from build123d import *

# Parameters (mm, degrees)
CHAMFER_1_SIZE         = 0.5
EXTRUDE_1649_DEPTH     = 5.5
SKETCH_6_R             = 8
CUT_EXTRUDE_1797_DEPTH = 0.5
SKETCH_9_R             = 2.5
EXTRUDE_1978_DEPTH     = 3
HOLE_WIZARD_M2_5_D     = 2.5


with BuildPart() as part:
    # Эскиз2 → Revolve 1260 (revolve)
    with BuildSketch(Plane.XY):
        Polygon((0, 4.5), (-9.5, 4.5), (-9.5, -1.5), (-6, -1.5), (-6, 0), (0, 0), align=None)
    revolve(axis=Axis((0, 4.5, 0), (0, -1, 0)))

    # Фаска1
    chamfer_1_edges = [part.edges().sort_by_distance(p)[0] for p in [
        (9.5, 4.5, 0),
    ]]
    chamfer(chamfer_1_edges, length=CHAMFER_1_SIZE)

    # Эскиз8 → Extrude 1649 (add)
    with BuildSketch(Plane.XZ):
        with BuildLine():
            Line((-1.175, 3.175), (1.175, 3.175))
            ThreePointArc((1.175, 3.175), (2.589213562, 2.589213562), (3.175, 1.175))
            Line((3.175, 1.175), (3.175, -1.175))
            ThreePointArc((3.175, -1.175), (2.589213562, -2.589213562), (1.175, -3.175))
            Line((1.175, -3.175), (-1.175, -3.175))
            ThreePointArc((-1.175, -3.175), (-2.589213562, -2.589213562), (-3.175, -1.175))
            Line((-3.175, -1.175), (-3.175, 1.175))
            ThreePointArc((-3.175, 1.175), (-2.589213562, 2.589213562), (-1.175, 3.175))
        make_face()
    extrude(amount=EXTRUDE_1649_DEPTH)

    # Эскиз6 → Cut-Extrude 1797 (cut)
    with BuildSketch(Plane(origin=(0, 4.5, 0), x_dir=(1, 0, 0), z_dir=(0, 1, 0))):
        with Locations(Location((0, 0, 0), (0, 0, 180))):
            Circle(SKETCH_6_R)
    extrude(amount=-CUT_EXTRUDE_1797_DEPTH, mode=Mode.SUBTRACT)

    # Эскиз9 → Extrude 1978 (add)
    with BuildSketch(Plane.XZ.offset(5.5)):
        Circle(SKETCH_9_R)
    extrude(amount=EXTRUDE_1978_DEPTH)

    # Отверстие M2,5 (through all)
    with Locations(Plane(origin=(0, -8.5, 0), x_dir=(-1, 0, 0), z_dir=(0, -1, 0))):
        with Locations((0, 0)):
            Hole(HOLE_WIZARD_M2_5_D / 2)


solid = part.part
The listing builds one solid part. Answer for the finished solid, in the listing's coordinates (mm). A direction names the side the tool comes from. Round coordinates to 2 decimals unless told otherwise and drop trailing zeros. Order: outer loops, then holes, each group sorted by start corner. A loop starts at its lowest first (then second) coordinate and runs counter-clockwise, first axis right, second up. Notation, with made-up numbers: (37, -9.75) -> (88, -9.75) arc R36 cw to (88, 28.25) -> close; hole circle Ø8 at (-16, 57). An arc over 180 degrees is marked (long way). Write each question's results on one line, items separated by ' | '. Start each with the question number.
Q1. Find section D-D (y = -3.5). Determine the outline of the cut face in (x, z) (3 decimals), then the cut area to 3 significant figures.
Q2. Find section B-B (x = 0). Determine the outline of the cut face in (y, z) (3 decimals).
Q3. Straight lines are drawn through the part: probe 1 along Z at (x, y) = (0, -0.75) (3 decimals); probe 2 along Z at (x, y) = (0, -2.25) (3 decimals); probe 3 along Y at (x, z) = (-6.25, -1). For each, find the intervals that lie inside material, in ascending order. Write a range as from..to.
Q4. Find section C-C (z = 0). Determine the outline of the cut face in (x, y) (3 decimals).
Q5. Find section A-A (y = -1). Determine the outline of the cut face in (x, z) (3 decimals), then the cut area to 3 significant figures.
Q6. The mould has two halves that part along X. Classify faces 4 (the cylindrical face through (2.605, -2.712, -2.574)), 5 (the flat face through (0, -3, 3.175)), 6 (the flat face through (-1, -8.5, -1)), 7 (the cylindrical face through (-4.38, 1.21, 8.43)): pulls with the +X half, pulls with the -X half, needs draft (parallel to the pull), parting line crosses it, or undercut.
Q7. Which of the six approach directions +Z, -Z, +X, -X, +Y, -Y give full straight-line access (tool end or side, diameter ignored) to faces 1 (the cylindrical face through (-0.27, -2.16, 1.22)), 2 (the flat face through (0.1, -1.5, 6.2)), 3 (the flat face through (-2, 4, 0))?
Q8. Each of these flat-tipped pins is pushed along its axis until it touches: pin 1 (1 mm diameter, centred on x = 4.5, y = -6.5, fed in from -Z); pin 2 (5 mm diameter, centred on x = 1.5, z = 3.5, fed in from +Y); pin 3 (10 mm diameter, centred on x = -7, z = 3, fed in from -Y). Where does it stop, or does it pass through?
Worked answers:
1) outline: (-3.175, -1.175) arc R2 ccw to (-1.175, -3.175) -> (1.175, -3.175) arc R2 ccw to (3.175, -1.175) -> (3.175, 1.175) arc R2 ccw to (1.175, 3.175) -> (-1.175, 3.175) arc R2 ccw to (-3.175, 1.175) -> close; hole circle Ø2.5 at (0, 0) | area: 32.0 mm2
2) outline: (-8.5, -2.5) -> (-5.5, -2.5) -> (-5.5, -3.175) -> (0, -3.175) -> (0, -6) -> (-1.5, -6) -> (-1.5, -9.5) -> (4, -9.5) -> (4.5, -9) -> (4.5, -8) -> (4, -8) -> (4, -1.25) -> (-8.5, -1.25) -> close; (-8.5, 1.25) -> (4, 1.25) -> (4, 8) -> (4.5, 8) -> (4.5, 9) -> (4, 9.5) -> (-1.5, 9.5) -> (-1.5, 6) -> (0, 6) -> (0, 3.175) -> (-5.5, 3.175) -> (-5.5, 2.5) -> (-8.5, 2.5) -> close
3) probe 1: z = -9.5..-6, -3.175..-1.25, 1.25..3.175, 6..9.5 | probe 2: z = -3.175..-1.25, 1.25..3.175 | probe 3: y = -1.5..4
4) outline: (-9.5, -1.5) -> (-6, -1.5) -> (-6, 0) -> (-3.175, 0) -> (-3.175, -5.5) -> (-2.5, -5.5) -> (-2.5, -8.5) -> (-1.25, -8.5) -> (-1.25, 4) -> (-8, 4) -> (-8, 4.5) -> (-9, 4.5) -> (-9.5, 4) -> close; (1.25, -8.5) -> (2.5, -8.5) -> (2.5, -5.5) -> (3.175, -5.5) -> (3.175, 0) -> (6, 0) -> (6, -1.5) -> (9.5, -1.5) -> (9.5, 4) -> (9, 4.5) -> (8, 4.5) -> (8, 4) -> (1.25, 4) -> close
5) outline: circle Ø19 at (0, 0); (-3.175, -1.175) arc R2 ccw to (-1.175, -3.175) -> (1.175, -3.175) arc R2 ccw to (3.175, -1.175) -> (3.175, 1.175) arc R2 ccw to (1.175, 3.175) -> (-1.175, 3.175) arc R2 ccw to (-3.175, 1.175) -> close; hole circle Ø12 at (0, 0); hole circle Ø2.5 at (0, 0) | area: 202 mm2
6) face 4: undercut | face 5: undercut | face 6: needs draft | face 7: parting line crosses it
7) face 1: +Y, -Y | face 2: -Y | face 3: +Y
8) pin 1: passes through | pin 2: stops at y = 4 | pin 3: stops at y = -5.5
